Could you check a few things on this drawing? It's one solid part, dimensions in mm from its lowest x, y, z. Give positions to 0.01 mm unless a question says otherwise; leave off trailing zeros. Order: outer loops, then holes, each group sorted by start corner. A loop starts at its lowest first (then second) coordinate and runs counter-clockwise, first axis right, second up. Notation, with made-up numbers: (44.5, 34) -> (69.5, 34) arc R6 ccw to (69.5, 38) -> close; hole circle Ø4 at (69, 56). An arc over 180 degrees is marked (long way). Use one line per item in the form item = value. Start each with the question number.
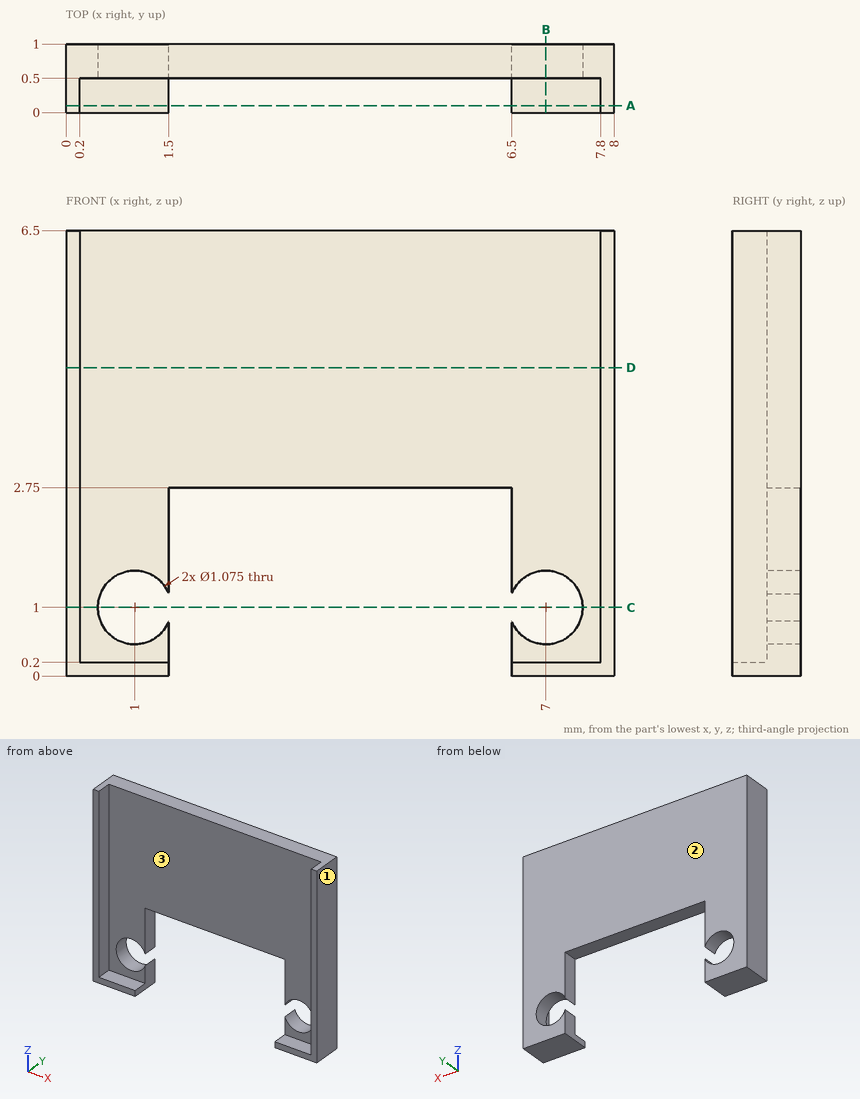
(1) I'm going to push a flat-ended pin straight in: pin 1 Ø1.9 at (x, z) = (2.5, 4.5) entering from -Y. Where does the tip first touch, or does it pass through?
(2) Imagine slicing it at B-B (x = 7). Write out the boundary of the cut face in (y, z), plus the area to 3 significant figures.
(3) Imagine slicing it at A-A (y = 0.1). Write out the boundary of the cut face in (x, z).
(4) Imagine slicing it at C-C (z = 1). Write out the boundary of the cut face in (x, y).
(5) Please list where these lines run through material, in increasing order: probe 1 along X at (y, z) = (0.45, 2.5); probe 2 along X at (y, z) = (0.8, 1); probe 3 along Z at (x, y) = (1, 0.7).
(6) Imagine slicing it at D-D (z = 4.5). Write out the boundary of the cut face in (x, y), plus the area to 3 significant figures.
(7) We'd pull the mould along X, two halves only. Please class the marked faces 1, 2 and 3: pulls with the +X half, pulls with the -X half, needs draft (parallel to the pull), parting line crosses it, or undercut.
Calculated:
q1.pin_1 = 0.5
q2.outline = (0, 0) -> (1, 0) -> (1, 0.46) -> (0.5, 0.46) -> (0.5, 0.2) -> (0, 0.2) -> close; (0.5, 1.54) -> (1, 1.54) -> (1, 6.5) -> (0.5, 6.5) -> close
q2.area = 2.81 mm2
q3.outline = (0, 0) -> (1.5, 0) -> (1.5, 0.2) -> (0.2, 0.2) -> (0.2, 6.5) -> (0, 6.5) -> close; (6.5, 0) -> (8, 0) -> (8, 6.5) -> (7.8, 6.5) -> (7.8, 0.2) -> (6.5, 0.2) -> close
q4.outline = (0, 0) -> (0.2, 0) -> (0.2, 0.5) -> (0.46, 0.5) -> (0.46, 1) -> (0, 1) -> close; (7.54, 0.5) -> (7.8, 0.5) -> (7.8, 0) -> (8, 0) -> (8, 1) -> (7.54, 1) -> close
q5.probe_1 = 0 to 0.2, 7.8 to 8
q5.probe_2 = 0 to 0.46, 7.54 to 8
q5.probe_3 = 0 to 0.46, 1.54 to 6.5
q6.outline = (0, 0) -> (0.2, 0) -> (0.2, 0.5) -> (7.8, 0.5) -> (7.8, 0) -> (8, 0) -> (8, 1) -> (0, 1) -> close
q6.area = 4.20 mm2
q7.face_1 = pulls with the +X half
q7.face_2 = needs draft
q7.face_3 = undercut
